The model under review builds one solid part; all positions refer to its coordinate system, in mm. A direction names the side the tool comes from. Give positions to 0.01 mm unless a question says otherwise; leave off trailing zeros. Order: outer loops, then holes, each group sorted by start corner. A loop starts at its lowest first (then second) coordinate and runs counter-clockwise, first axis right, second up. Notation, with made-up numbers: (8, -28) -> (55, -28) arc R18 ccw to (55, -17) -> close; hole circle Ø8 at (-17, 66). An arc over 180 degrees is marked (long way). Use one line per item in the form item = value.
```python
from build123d import *


# Not quite as in the source:
# - a fillet or chamfer that OpenCascade refuses, or shapes differently, is made with other operations: its cross-section is extruded or revolved along the edge and cut away or added


with BuildPart() as f1:
    # F0 (on Front) → F1 (revolve)
    with BuildSketch(Plane.XZ):
        Polygon((25.4, -69.85), (25.4, 69.85), (14.1084063798, 69.85), (14.1084063798, 79.8223763704), (11.0044367611, 79.8223763704), (11.0044367611, 75.8906826377), (11.0044367611, 64.0955939889), (22.3856568336, 64.0955939889), (22.3856568336, -66.8919235468), (1.6925277887, -66.8919235468), (3.1410455704, 75.8906826377), (3.1410455704, 79.8223763704), (0, 79.8223763704), (0, 0), (0, -69.85), align=None)
    revolve(axis=Axis((0, 0, 39.9111881852), (0, 0, -1)))

    # F2: fillet of radius 5.08 on 2 edges, made by hand

    # F2_s1 → F2_t2 (revolve, cut)
    with BuildSketch(Plane.XZ):
        with BuildLine():
            ThreePointArc((25.4004, 64.7690343146), (23.9121024484, 68.3621024484), (20.3190343146, 69.8504))
            Line((20.3190343146, 69.8504), (20.3190343146, 70.3585365685))
            ThreePointArc((20.3190343146, 70.3585365685), (22.8595171573, 70.3581365685), (25.4, 70.3581365685))
            Line((25.4, 70.3581365685), (25.9081365685, 69.85))
            ThreePointArc((25.9081365685, 69.85), (25.9081365685, 67.3095171573), (25.9085365685, 64.7690343146))
            Line((25.9085365685, 64.7690343146), (25.4004, 64.7690343146))
        make_face()
    revolve(axis=Axis((0, 0, 69.85), (0, 0, -1)), mode=Mode.SUBTRACT)

    # F2_s3 → F2_t4 (revolve, cut)
    with BuildSketch(Plane.XZ):
        with BuildLine():
            ThreePointArc((14.1088063798, 75.1418102884), (13.2622316021, 77.9501591266), (11.0045924005, 79.8227448489))
            Line((11.0045924005, 79.8227448489), (11.2023075712, 80.2908383049))
            ThreePointArc((11.2023075712, 80.2908383049), (12.5564993902, 80.330512939), (14.1084063798, 80.330512939))
            Line((14.1084063798, 80.330512939), (14.6165429484, 79.8223763704))
            ThreePointArc((14.6165429484, 79.8223763704), (14.6165429484, 77.4820933294), (14.6169429484, 75.1418102884))
            Line((14.6169429484, 75.1418102884), (14.1088063798, 75.1418102884))
        make_face()
    revolve(axis=Axis((0, 0, 79.8223763704), (0, 0, -1)), mode=Mode.SUBTRACT)


solid = f1.part
```
1. Add section B-B on z = -22.5. Give the boundary of the cut face in (x, y), then the cut area to 3 significant figures.
Values:
outline = circle Ø50.8 at (0, 0); circle Ø4.29 at (0, 0); hole circle Ø44.77 at (0, 0)
area = 467 mm^2
2. For L1, parallel to Y at x = 0, z = 74.25; L2, parallel to Z at x = -16, y = -8.5; L3, parallel to X at y = 0, z = -22.5, list the stretches that pass through material, from the lowest coordinate up.
Values:
L1 = -14.11 to -11, -3.12 to 3.12, 11 to 14.11
L2 = -69.85 to -66.89, 64.1 to 69.85
L3 = -25.4 to -22.39, -2.14 to 2.14, 22.39 to 25.4
3. Tool access review of faces 1 (the face through (4, -14, 69.85)), 2 (the face through (-5, -10, 64.096)), 3 (the face through (-5.506, 24.796, -1.566)): name each direction out of +Z, -Z, +X, -X, +Y, -Y from which nothing blocks a thin tool from reaching the whole face with its end or side.
Values:
face_1 = +Z
face_2 = none
face_3 = +Z, -Z
4. The part is to be moulded in two halves that separate along X. For faces 4 (the face through (7.58, -11.9, 72.57)), 5 (the face through (-1.79, -1.64, 5.5)), 6 (the face through (0, 0, 79.822)), say which applies: +X half, -X half, draft (parallel to the pull), parting line (faces both ways), or undercut.
Values:
face_4 = parting line
face_5 = undercut
face_6 = draft
5. For pin 1 Ø5 at (x, z) = (-16.5, -32.5) entering from +Y; pin 2 Ø10 at (y, z) = (19, 36.5) entering from -X; pin 3 Ø12 at (x, z) = (-20.5, 44) entering from -Y; pin 4 Ø6 at (y, z) = (-1.5, 50.5) entering from -X, all flat-tipped, find the tip position at first contact; note any pin that passes through.
Values:
pin_1 = 21.19
pin_2 = -21.19
pin_3 = -20.85
pin_4 = -25.4
6. Add section A-A on z = 31.5. Give the boundary of the cut face in (x, y).
Values:
outline = circle Ø50.8 at (0, 0); circle Ø5.38 at (0, 0); hole circle Ø44.77 at (0, 0)
